Can you work these out from the model? Positions are in its coordinate system, mm. A direction names the side the tool comes from. Give positions to 0.01 mm unless a question says otherwise; leave off trailing zeros. Loops run counter-clockwise (first coordinate to the right, second up) from the corner with the lowest first, then second, coordinate; pieces in that order, holes last. Notation, with made-up numbers: (22.25, 36) -> (31.25, 36) arc R25 ccw to (31.25, 74) -> close; hole circle Ø3 at (42, 86). An arc over 180 degrees is marked (long way). One line per question, with ' | ' between items.
from build123d import *

# Parameters (mm, degrees)
EXTRUDE1_DEPTH   = 12
F_2_STK_M6_D     = 5
F_2_STK_M6_DEPTH = 14
F_2_STK_M6_TIP   = 1.502151548


with BuildPart() as part:
    # Sketch1 → Extrude1 (new body)
    with BuildSketch(Plane.XY):
        with BuildLine():
            Line((-6.785898385, 0), (6.785898385, 0))
            ThreePointArc((6.785898385, 0), (7.785898385, -0.267949192), (8.517949192, -1))
            ThreePointArc((8.517949192, -1), (10.76763809, -1.931851653), (12.25, 0))
            Line((12.25, 0), (12.25, 43))
            ThreePointArc((12.25, 43), (12.542893219, 43.707106781), (13.25, 44))
            Line((13.25, 44), (35, 44))
            ThreePointArc((35, 44), (38.535533906, 42.535533906), (40, 39))
            Line((40, 39), (40, -7.783053374))
            ThreePointArc((40, -7.783053374), (40.237039929, -9.947449513), (40.93692213, -12.009235991))
            Line((40.93692213, -12.009235991), (68.553018239, -71.232145215))
            ThreePointArc((68.553018239, -71.232145215), (68.364269215, -74.111898825), (65.834094878, -75.5))
            Line((65.834094878, -75.5), (5.547687523, -75.5))
            ThreePointArc((5.547687523, -75.5), (3.880976824, -74.994408837), (2.776048925, -73.648050297))
            Line((2.776048925, -73.648050297), (-9.873472677, -43.109403687))
            ThreePointArc((-9.873472677, -43.109403687), (-10.389591852, -42.279416539), (-11.145111274, -41.659377773))
            Line((-11.145111274, -41.659377773), (-35, -27.886751346))
            ThreePointArc((-35, -27.886751346), (-38.660254038, -24.226497308), (-40, -19.226497308))
            Line((-40, -19.226497308), (-40, 39))
            ThreePointArc((-40, 39), (-38.535533906, 42.535533906), (-35, 44))
            Line((-35, 44), (-13.25, 44))
            ThreePointArc((-13.25, 44), (-12.542893219, 43.707106781), (-12.25, 43))
            Line((-12.25, 43), (-12.25, 0))
            ThreePointArc((-12.25, 0), (-10.76763809, -1.931851653), (-8.517949192, -1))
            ThreePointArc((-8.517949192, -1), (-7.785898385, -0.267949192), (-6.785898385, 0))
        make_face()
    extrude(amount=EXTRUDE1_DEPTH)

    # 2 stk M6
    with Locations(Plane(origin=(0, 44, 0), x_dir=(-1, 0, 0), z_dir=(0, 1, 0))):
        with Locations((-22, 6), (22, 6)):
            Hole(F_2_STK_M6_D / 2, depth=F_2_STK_M6_DEPTH)
            with Locations((0, 0, -(F_2_STK_M6_DEPTH + F_2_STK_M6_TIP / 2))):  # 118° drill point
                Cone(0, F_2_STK_M6_D / 2, F_2_STK_M6_TIP, mode=Mode.SUBTRACT)


solid = part.part
Q1. If we section it at A-A (y = 33.5): Write out the boundary of the cut face in (x, z).
Entries:
outline: (-40, 0) -> (-12.25, 0) -> (-12.25, 12) -> (-40, 12) -> close; (12.25, 0) -> (40, 0) -> (40, 12) -> (12.25, 12) -> close; hole circle Ø5 at (-22, 6); hole circle Ø5 at (22, 6)
Q2. If we section it at C-C (z = 10): Write out the boundary of the cut face in (x, y), plus the area to 3 significant figures.
Entries:
outline: (-40, -19.23) arc R10 ccw to (-35, -27.89) -> (-11.15, -41.66) arc R3 cw to (-9.87, -43.11) -> (2.78, -73.65) arc R3 ccw to (5.55, -75.5) -> (65.83, -75.5) arc R3 ccw to (68.55, -71.23) -> (40.94, -12.01) arc R10 cw to (40, -7.78) -> (40, 39) arc R5 ccw to (35, 44) -> (13.25, 44) arc R1 ccw to (12.25, 43) -> (12.25, 0) arc R2 cw to (8.52, -1) arc R2 ccw to (6.79, 0) -> (-6.79, 0) arc R2 ccw to (-8.52, -1) arc R2 cw to (-12.25, 0) -> (-12.25, 43) arc R1 ccw to (-13.25, 44) -> (-35, 44) arc R5 ccw to (-40, 39) -> close | area: 7,970 mm²
Q3. On a 3-axis mill with a long thin cutter (end or side, diameter ignored), from which of +Z, -Z, +X, -X, +Y, -Y can I reach the whole of each face in a straight line? I mean faces 4 (the face through (40, 16, 6)), 5 (the face through (19.5, 36.9, 6.1)), 6 (the face through (-38.623, -24.29, 5.916)), 7 (the face through (12.25, 21, 6)). Say none if no direction works.
Entries:
face 4: +Z, -Z, +X, +Y | face 5: +Y | face 6: +Z, -Z, -X, -Y | face 7: +Z, -Z, +Y
Q4. If I drill on probe 1 along X at (y, z) = (38, 6); probe 2 along Z at (x, y) = (-22, 35); probe 3 along X at (y, z) = (11.5, 9), over which ranges is the centre line in solid material (lowest first)? Write a range as from..to.
Entries:
probe 1: -40..-24.5, -19.5..-12.25, 12.25..19.5, 24.5..40 | probe 2: 0..3.5, 8.5..12 | probe 3: -40..-12.25, 12.25..40
Q5. If we section it at B-B (y = 18.5): Write out the boundary of the cut face in (x, z).
Entries:
outline: (-40, 0) -> (-12.25, 0) -> (-12.25, 12) -> (-40, 12) -> close; (12.25, 0) -> (40, 0) -> (40, 12) -> (12.25, 12) -> close
Q6. For pin 1 Ø6 at (y, z) = (21, 4.5) entering from +X; pin 2 Ø3.5 at (x, z) = (0.5, 7) entering from +Y; pin 3 Ø2 at (y, z) = (-40.5, 6.5) entering from +X, each with a flat end and sliding along its axis, tell me the tip position at first contact or that it passes through.
Entries:
pin 1: x = 40 | pin 2: y = 0 | pin 3: x = 54.69
Q7. If we section it at D-D (x = 62): Write out the boundary of the cut face in (y, z).
Entries:
outline: (-75.5, 0) -> (-57.18, 0) -> (-57.18, 12) -> (-75.5, 12) -> close
Q8. If we mould it in two halves opening along Z, with no side actions, what happens to faces 1 (the face through (15, -15, 12)), 2 (the face through (40.23, -9.92, 5.92)), 3 (the face through (21.6, 28.76, 5.83))? For each: pulls with the +Z half, pulls with the -Z half, needs draft (parallel to the pull), parting line crosses it, or undercut.
Entries:
face 1: pulls with the +Z half | face 2: needs draft | face 3: undercut
